```python
from build123d import *

# Parameters (mm, degrees)
SKETCH_R   = 26.5
SKETCH_R_2 = 4
PAD_DEPTH  = 1
FILLET_R   = 40


with BuildPart() as part:
    # Sketch → Pad (new body, symmetric)
    with BuildSketch(Plane.XY):
        with BuildLine():
            ThreePointArc((5.368922, 43.930824), (0, 46), (-5.368922, 43.930824))
            Line((-32.908965, 19), (-5.368922, 43.930824))
            Line((-32.908965, 19), (-40.729671, -17.315789))
            ThreePointArc((-40.729671, -17.315789), (-39.837169, -23), (-35.360749, -26.615035))
            Line((-35.360749, -26.615035), (0, -38))
            Line((0, -38), (35.360749, -26.615035))
            ThreePointArc((35.360749, -26.615035), (39.837169, -23), (40.729671, -17.315789))
            Line((32.908965, 19), (40.729671, -17.315789))
            Line((32.908965, 19), (5.368922, 43.930824))
        make_face()
        Circle(SKETCH_R, mode=Mode.SUBTRACT)
        with Locations((0, 38)):
            Circle(SKETCH_R_2, mode=Mode.SUBTRACT)
        with Locations((32.908965, -19)):
            Circle(SKETCH_R_2, mode=Mode.SUBTRACT)
        with Locations((-32.908965, -19)):
            Circle(SKETCH_R_2, mode=Mode.SUBTRACT)
    extrude(amount=PAD_DEPTH, both=True)

    # Fillet
    fillet_edges = [part.edges().sort_by_distance(p)[0] for p in [
        (32.908965, 19, 0),
        (0, -38, 0),
        (-32.908965, 19, 0),
    ]]
    fillet(fillet_edges, radius=FILLET_R)


solid = part.part
```
Model file for the job. Use its own axes, mm. Give positions to 0.01 mm unless a question says otherwise; leave off trailing zeros. Loops run counter-clockwise (first coordinate to the right, second up) from the corner with the lowest first, then second, coordinate; pieces in that order, holes last. Notation, with made-up numbers: (-24.75, 17) -> (-11.75, 17) arc R6 ccw to (-11.75, 23) -> close; hole circle Ø11 at (-3.5, 72.5). An arc over 180 degrees is marked (long way). Write each question's results on one line, items separated by ' | '.
(1) Cut at B-B on y = -19. List the corners of the cut face in (x, z).
Geometry results:
outline: (-40.91, -1) -> (-36.91, -1) -> (-36.91, 1) -> (-40.91, 1) -> close; (-28.91, -1) -> (-18.47, -1) -> (-18.47, 1) -> (-28.91, 1) -> close; (18.47, -1) -> (28.91, -1) -> (28.91, 1) -> (18.47, 1) -> close; (36.91, -1) -> (40.91, -1) -> (40.91, 1) -> (36.91, 1) -> close
(2) Cut at C-C on x = 0. List the corners of the cut face in (y, z), and give its area (3 significant figures).
Geometry results:
outline: (-35.98, -1) -> (-26.5, -1) -> (-26.5, 1) -> (-35.98, 1) -> close; (26.5, -1) -> (34, -1) -> (34, 1) -> (26.5, 1) -> close; (42, -1) -> (46, -1) -> (46, 1) -> (42, 1) -> close | area: 42.0 mm²
(3) Pull direction Y, two halves, no side cores. Call faces 1 (the flat face through (14.491, 35.673, 0.014)), 2 (the cylindrical face through (14.246, 22.345, -0.014)), 3 (the cylindrical face through (-0.521, 41.966, -0.014)), 4 (the flat face through (18, -22, -1)): released by +Y, released by -Y, zero draft, split by the parting line, or undercut.
Geometry results:
face 1: released by +Y | face 2: undercut | face 3: undercut | face 4: zero draft
(4) Probe line 1 along Y through (x, z) = (-3.5, 0); line 2 along Y through (x, z) = (-20.5, 0.3); line 3 along Y through (x, z) = (-24.5, -0.9). List the from-to ranges inside material, lowest first.
Geometry results:
line 1: y = -35.82 to -26.27, 26.27 to 36.06, 39.94 to 45.19 | line 2: y = -31.4 to -16.79, 16.79 to 30.23 | line 3: y = -30.11 to -10.1, 10.1 to 26.57
(5) Flat gauge pin, fed straight in: pin 1 Ø10.5 at (x, y) = (-32.91, -19) entering from +Z. Where does the tip first touch, or does it go through?
Geometry results:
pin 1: stops at z = 1
(6) Cut at A-A on z = -0.1. List the corners of the cut face in (x, y), and give its area (3 significant figures).
Geometry results:
outline: (-40.73, -17.32) arc R8 ccw to (-35.36, -26.62) -> (-12.26, -34.05) arc R40 ccw to (12.26, -34.05) -> (35.36, -26.62) arc R8 ccw to (40.73, -17.32) -> (35.62, 6.41) arc R40 ccw to (23.36, 27.64) -> (5.37, 43.93) arc R8 ccw to (-5.37, 43.93) -> (-23.36, 27.64) arc R40 ccw to (-35.62, 6.41) -> close; hole circle Ø8 at (-32.91, -19); hole circle Ø53 at (0, 0); hole circle Ø8 at (0, 38); hole circle Ø8 at (32.91, -19) | area: 2,380 mm²
(7) Cut at D-D on y = 38. List the corners of the cut face in (x, z), and give its area (3 significant figures).
Geometry results:
outline: (-11.92, -1) -> (-4, -1) -> (-4, 1) -> (-11.92, 1) -> close; (4, -1) -> (11.92, -1) -> (11.92, 1) -> (4, 1) -> close | area: 31.7 mm²
